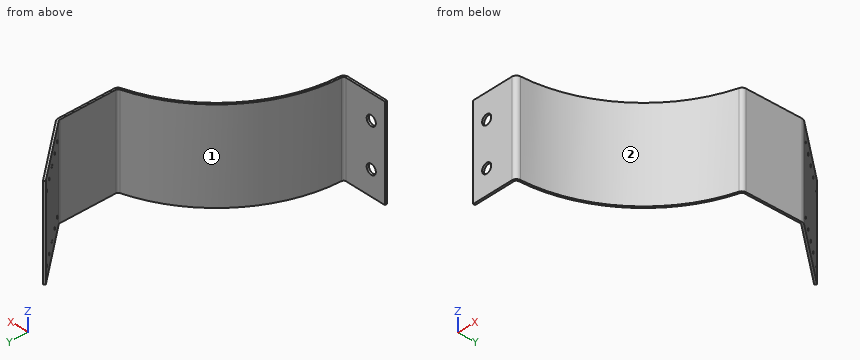
from build123d import *

# Parameters (mm, degrees)
BASE_FLANGE1_DEPTH           = 119.6975
EDGE_FLANGE1_DEPTH           = 119.6975
EDGE_FLANGE2_STRIP_CUT_DEPTH = 119.6975
EDGE_FLANGE2_DEPTH           = 119.6975
EDGE_FLANGE3_DEPTH           = 119.6975
SKETCH20_R                   = 6.35
CUT_EXTRUDE1_DEPTH           = 2.65684
SKETCH21_R                   = 2.032
CUT_EXTRUDE2_DEPTH           = 2.65684


# Sheet-metal steps are written as plain solids
with BuildPart() as part:
    # Sketch1 → Base-Flange1 (new body)
    with BuildSketch(Plane.XY):
        with BuildLine():
            ThreePointArc((-50.8, 170.388379885), (-140.856418383, 108.500273734), (-177.710803869, 5.63118))
            Line((-177.710803869, 5.63118), (-180.366311024, 5.715325918))
            ThreePointArc((-180.366311024, 5.715325918), (-142.961215721, 110.121577824), (-51.559097143, 172.934469105))
            Line((-51.559097143, 172.934469105), (-50.8, 170.388379885))
        make_face()
    extrude(amount=BASE_FLANGE1_DEPTH)

    # Edge-Flange1 section (across the edge) → Edge-Flange1 (add)
    with BuildSketch(Plane(origin=(-49.291175996, 173.610632552, 119.6975), x_dir=(-0.9999999996342678, -2.7045604981568168e-05, 0), z_dir=(0, 0, -1))):
        with BuildLine():
            Line((-2.65684, 2.366572064), (-2.65684, 76.2))
            Line((-2.65684, 76.2), (0, 76.2))
            Line((0, 76.2), (0, 2.366572064))
            ThreePointArc((0, 2.366572064), (0.62936233, 0.469112223), (2.267939433, -0.676102109))
            Line((2.267939433, -0.676102109), (1.508911151, -3.222211858))
            ThreePointArc((1.508911151, -3.222211858), (-1.500827273, -1.118682173), (-2.65684, 2.366572064))
        make_face()
    extrude(amount=EDGE_FLANGE1_DEPTH)

    # Edge-Flange2 strip (across the edge) → Edge-Flange2 strip cut (cut)
    with BuildSketch(Plane(origin=(-49.293236871, 249.810632524, 119.6975), x_dir=(-0.7660270582590358, -0.6428083275868537, 0), z_dir=(0, 0, -1))):
        Polygon((-12.205285278, 10.412383287), (-1.292448625, -2.593029), (0.742808893, -0.885245167), (-10.17002776, 12.12016712), align=None)
    extrude(amount=EDGE_FLANGE2_STRIP_CUT_DEPTH, mode=Mode.SUBTRACT)

    # Edge-Flange2 section (across the edge) → Edge-Flange2 (add)
    with BuildSketch(Plane(origin=(-49.293236871, 249.810632524, 119.6975), x_dir=(-0.7660270582590358, -0.6428083275868537, 0), z_dir=(0, 0, -1))):
        with BuildLine():
            Line((-2.65684, 1.155605494), (-2.65684, 101.6))
            Line((-2.65684, 101.6), (0, 101.6))
            Line((0, 101.6), (0, 1.155605494))
            ThreePointArc((0, 1.155605494), (0.191475929, 0.069691539), (0.742808893, -0.885245167))
            Line((0.742808893, -0.885245167), (-1.292448625, -2.593029))
            ThreePointArc((-1.292448625, -2.593029), (-2.305137014, -0.839001259), (-2.65684, 1.155605494))
        make_face()
    extrude(amount=EDGE_FLANGE2_DEPTH)

    # Edge-Flange3 section (across the edge) → Edge-Flange3 (add)
    with BuildSketch(Plane(origin=(-180.463740314, 2.640617339, 0), x_dir=(8.626632785421055e-05, 0.9999999962790604, 0), z_dir=(0, 0, 1))):
        with BuildLine():
            Line((-2.65684, 3.076251829), (-2.65684, 57.15))
            Line((-2.65684, 57.15), (0, 57.15))
            Line((0, 57.15), (0, 3.076251829))
            ThreePointArc((0, 3.076251829), (0.894756196, 0.86692768), (3.074716973, -0.097164046))
            Line((3.074716973, -0.097164046), (2.990800136, -2.75267845))
            ThreePointArc((2.990800136, -2.75267845), (-1.013351819, -0.981834768), (-2.65684, 3.076251829))
        make_face()
    extrude(amount=EDGE_FLANGE3_DEPTH)

    # Sketch20 → Cut-Extrude1 (cut)
    with BuildSketch(Plane(origin=(0.000226453, 2.625049375, 0), x_dir=(0.9999999962790604, -8.626632785420363e-05, 0), z_dir=(8.626632785420363e-05, 0.9999999962790604, 0))):
        with Locations(Location((-218.563967439, -31.75, 0), (0, 0, 180))):
            Circle(SKETCH20_R)
        with Locations(Location((-218.563967439, -87.9475, 0), (0, 0, 180))):
            Circle(SKETCH20_R)
    extrude(amount=-CUT_EXTRUDE1_DEPTH, mode=Mode.SUBTRACT)

    # Sketch21 → Cut-Extrude2 (cut)
    with BuildSketch(Plane(origin=(94.083750988, 78.949976994, 0), x_dir=(0, 0, 1), z_dir=(-0.7660270582590358, -0.6428083275868537, 0))):
        with Locations(Location((103.30434, 317.017474478, 0), (0, 0, 270))):
            Circle(SKETCH21_R)
        with Locations(Location((103.30434, 296.697474478, 0), (0, 0, 270))):
            Circle(SKETCH21_R)
        with Locations(Location((103.30434, 276.377474478, 0), (0, 0, 270))):
            Circle(SKETCH21_R)
        with Locations(Location((103.30434, 256.057474478, 0), (0, 0, 270))):
            Circle(SKETCH21_R)
        with Locations(Location((103.30434, 235.737474478, 0), (0, 0, 270))):
            Circle(SKETCH21_R)
        with Locations(Location((16.39316, 235.737474478, 0), (0, 0, 270))):
            Circle(SKETCH21_R)
        with Locations(Location((16.39316, 256.057474478, 0), (0, 0, 270))):
            Circle(SKETCH21_R)
        with Locations(Location((16.39316, 276.377474478, 0), (0, 0, 270))):
            Circle(SKETCH21_R)
        with Locations(Location((16.39316, 296.697474478, 0), (0, 0, 270))):
            Circle(SKETCH21_R)
        with Locations(Location((16.39316, 317.017474478, 0), (0, 0, 270))):
            Circle(SKETCH21_R)
    extrude(amount=-CUT_EXTRUDE2_DEPTH, mode=Mode.SUBTRACT)


solid = part.part
Check sheet for the modelled part. Datum: model origin and axes. Units: mm. Face numbers are marked on the shaded views. Round coordinates to 2 decimals unless told otherwise and drop trailing zeros. Loops run counter-clockwise (first coordinate to the right, second up) from the corner with the lowest first, then second, coordinate; pieces in that order, holes last.
1. Mould release check, pull along Y, two halves, no side actions. Record for the marked faces 1 and 2: released by +Y, released by -Y, zero draft, split by the parting line, or undercut.
2. Scan lines: probe 1 along X at (y, z) = (211.5, 50); probe 2 along Y at (x, z) = (-88, 78); probe 3 along Y at (x, z) = (-65.5, 37.5). Record each from-to range of solid material in increasing order.
3. Sectioned sample at A-A on z = 31.75. Record the boundary of the cut face in (x, y) (3 decimals), and give its area (3 significant figures).
4. Sectioned sample at B-B on y = 28. Record the boundary of the cut face in (x, z), and give its area (3 significant figures).
5. Gauge pin test, flat ends, axial feed: pin 1 Ø2 at (x, z) = (-125.5, 14) entering from -Y; pin 2 Ø1 at (x, z) = (-211.5, 48.5) entering from +Y; pin 3 Ø10 at (y, z) = (148.5, 56.5) entering from +X; pin 4 Ø10 at (x, z) = (-218.56, 87.95) entering from +Y. Record the tip position at first contact, or that the pin passes through.
6. Sectioned sample at C-C on y = 230.5. Record the boundary of the cut face in (x, z).
Recorded:
1. face 1: undercut
1. face 2: released by -Y
2. probe 1: x = -49.29 to -46.64
2. probe 2: y = 154.5 to 157.55, 295.94 to 300.07
2. probe 3: y = 165.3 to 168.15, 269.12 to 273.26
3. outline: (-237.614, -0.011) - (-224.914, -0.012) - (-224.914, 2.644) - (-237.614, 2.646) - close; (-212.214, -0.013) - (-183.54, -0.016) arc R5.832 ccw to (-177.711, 5.631) arc R177.8 cw to (-50.8, 170.388) arc R5.832 ccw to (-46.634, 175.977) - (-46.636, 248.655) arc R5.832 ccw to (-48.001, 252.404) - (-112.567, 329.347) - (-114.603, 327.639) - (-50.036, 250.696) arc R3.175 cw to (-49.293, 248.655) - (-49.291, 175.977) arc R3.175 cw to (-51.559, 172.934) arc R180.457 ccw to (-180.366, 5.715) arc R3.175 cw to (-183.54, 2.641) - (-212.214, 2.643) - close
3. area: 1,210 mm2
4. outline: (-178.27, 0) - (-175.58, 0) - (-175.58, 119.7) - (-178.27, 119.7) - close
4. area: 322 mm2
5. pin 1: stops at y = 124.94
5. pin 2: stops at y = 2.64
5. pin 3: stops at x = -89.73
5. pin 4: passes through
6. outline: (-49.29, 0) - (-46.64, 0) - (-46.64, 119.7) - (-49.29, 119.7) - close
